from build123d import *

# Parameters (mm, degrees)
SKETCH_1_R          = 2
EXTRUDE_1_DEPTH     = 5
EXTRUDE_2_DEPTH     = 5
CUT_EXTRUDE_1_DEPTH = 6
EXTRUDE_3_DEPTH     = 5
FILLET_1_R          = 10
FILLET_2_R          = 2
SKETCH_6_R          = 2
CUT_EXTRUDE_2_DEPTH = 6


with BuildPart() as part:
    # 草图1 → 凸台-拉伸1 (new body)
    with BuildSketch(Plane(origin=(0, 0, 0), x_dir=(1, 0, 0), z_dir=(0, 1, 0))):
        with BuildLine():
            ThreePointArc((-20.0875, 4), (-23.044826598, 2.693365811), (-24.070081176, -0.372890305))
            ThreePointArc((-24.070081176, -0.372890305), (-22.780865811, -2.957326598), (-20.0875, -4))
            ThreePointArc((-20.0875, -4), (-17.130173402, -2.693365811), (-16.104918824, 0.372890305))
            Line((-16.104918824, 0.372890305), (-16.444526225, 4))
            Line((-16.444526225, 4), (-20.0875, 4))
        make_face()
        with Locations((-20.0875, 0)):
            Circle(SKETCH_1_R, mode=Mode.SUBTRACT)
        with BuildLine():
            Line((-27.14754486, 32.495352138), (-24.070081176, -0.372890305))
            ThreePointArc((-24.070081176, -0.372890305), (-23.044826598, 2.693365811), (-20.0875, 4))
            Line((-20.0875, 4), (-16.444526225, 4))
            Line((-16.444526225, 4), (-18.333300994, 24.172685504))
            Line((-18.333300994, 24.172685504), (-25.585127327, 29.683464909))
            ThreePointArc((-25.585127327, 29.683464909), (-26.661456606, 30.925425609), (-27.14754486, 32.495352138))
        make_face()
        with BuildLine():
            ThreePointArc((-20.74480004, 36.053019976), (-25.107780517, 36.364735365), (-27.14754486, 32.495352138))
            ThreePointArc((-27.14754486, 32.495352138), (-26.661456606, 30.925425609), (-25.585127327, 29.683464909))
            Line((-25.585127327, 29.683464909), (-18.333300994, 24.172685504))
            Line((-18.333300994, 24.172685504), (-19.182382508, 33.241132747))
            ThreePointArc((-19.182382508, 33.241132747), (-19.668470762, 34.811059276), (-20.74480004, 36.053019976))
        make_face()
        with Locations((-23.164963684, 32.868242443)):
            Circle(SKETCH_1_R, mode=Mode.SUBTRACT)
        with BuildLine():
            Line((22.507663644, 3.184777534), (-20.74480004, 36.053019976))
            ThreePointArc((-20.74480004, 36.053019976), (-19.668470762, 34.811059276), (-19.182382508, 33.241132747))
            Line((-19.182382508, 33.241132747), (-18.333300994, 24.172685504))
            Line((-18.333300994, 24.172685504), (8.212637649, 4))
            Line((8.212637649, 4), (20.0875, 4))
            ThreePointArc((20.0875, 4), (21.364388771, 3.790719598), (22.507663644, 3.184777534))
        make_face()
        with BuildLine():
            ThreePointArc((-16.104918824, 0.372890305), (-17.130173402, -2.693365811), (-20.0875, -4))
            Line((-20.0875, -4), (20.0875, -4))
            ThreePointArc((20.0875, -4), (18.810611229, -3.790719598), (17.667336356, -3.184777534))
            Line((17.667336356, -3.184777534), (8.212637649, 4))
            Line((8.212637649, 4), (-16.444526225, 4))
            Line((-16.444526225, 4), (-16.104918824, 0.372890305))
        make_face()
        with BuildLine():
            ThreePointArc((17.667336356, -3.184777534), (18.810611229, -3.790719598), (20.0875, -4))
            ThreePointArc((20.0875, -4), (23.878219598, -1.276888771), (22.507663644, 3.184777534))
            ThreePointArc((22.507663644, 3.184777534), (21.364388771, 3.790719598), (20.0875, 4))
            Line((20.0875, 4), (8.212637649, 4))
            Line((8.212637649, 4), (17.667336356, -3.184777534))
        make_face()
        with Locations((20.0875, 0)):
            Circle(SKETCH_1_R, mode=Mode.SUBTRACT)
        Polygon((-18.333300994, 24.172685504), (-16.444526225, 4), (8.212637649, 4), align=None)
    extrude(amount=EXTRUDE_1_DEPTH)

    # 草图2 → 凸台-拉伸2 (add)
    with BuildSketch(Plane(origin=(0, 5, 0), x_dir=(1, 0, 0), z_dir=(0, 1, 0))):
        with BuildLine():
            ThreePointArc((-20.0875, -4), (-22.780865811, -2.957326598), (-24.070081176, -0.372890305))
            Line((-24.070081176, -0.372890305), (-23.720962628, -4.10158193))
            ThreePointArc((-23.720962628, -4.10158193), (-22.290826699, -6.808468121), (-19.365512753, -7.711274824))
            Line((-19.365512753, -7.711274824), (20.460368699, -3.982583199))
            ThreePointArc((20.460368699, -3.982583199), (20.274137625, -3.995643427), (20.0875, -4))
            Line((20.0875, -4), (-20.0875, -4))
        make_face()
    extrude(amount=-EXTRUDE_2_DEPTH)

    # 草图3 → 切除-拉伸1 (cut, through all)
    with BuildSketch(Plane(origin=(0, 5, 0), x_dir=(1, 0, 0), z_dir=(0, 1, 0))):
        with BuildLine():
            ThreePointArc((-36.289327432, 17.433897667), (-37.629570165, 14.285674695), (-36.182704661, 11.185007239))
            ThreePointArc((-36.182704661, 11.185007239), (-31.653466249, 15.823666602), (-25.858788976, 18.731049718))
            Line((-25.858788976, 18.731049718), (-26.257218708, 22.986399698))
            ThreePointArc((-26.257218708, 22.986399698), (-31.612650276, 20.82332613), (-36.289327432, 17.433897667))
        make_face()
        with BuildLine():
            ThreePointArc((-25.858788976, 18.731049718), (-11.47348363, 17.605644606), (-1.756724615, 6.938492183))
            ThreePointArc((-1.756724615, 6.938492183), (0.40025314, 9.594618202), (-0.134776474, 12.974159854))
            ThreePointArc((-0.134776474, 12.974159854), (-11.569633945, 22.223545124), (-26.257218708, 22.986399698))
            Line((-26.257218708, 22.986399698), (-25.858788976, 18.731049718))
        make_face()
        with BuildLine():
            ThreePointArc((-7.176914189, 8.395044611), (-4.745829362, 6.62850376), (-1.756724615, 6.938492183))
            ThreePointArc((-1.756724615, 6.938492183), (-11.47348363, 17.605644606), (-25.858788976, 18.731049718))
            Line((-25.858788976, 18.731049718), (-25.456435977, 14.433798061))
            ThreePointArc((-25.456435977, 14.433798061), (-15.256790284, 14.622730376), (-7.176914189, 8.395044611))
        make_face()
        with BuildLine():
            ThreePointArc((-25.858788976, 18.731049718), (-31.653466249, 15.823666602), (-36.182704661, 11.185007239))
            ThreePointArc((-36.182704661, 11.185007239), (-33.358528619, 10.15793874), (-30.571035397, 11.280757314))
            ThreePointArc((-30.571035397, 11.280757314), (-28.168999159, 13.109133127), (-25.456435977, 14.433798061))
            Line((-25.456435977, 14.433798061), (-25.858788976, 18.731049718))
        make_face()
    extrude(amount=-CUT_EXTRUDE_1_DEPTH, mode=Mode.SUBTRACT)

    # 草图4 → 凸台-拉伸3 (add)
    with BuildSketch(Plane(origin=(0, 5, 0), x_dir=(1, 0, 0), z_dir=(0, 1, 0))):
        with BuildLine():
            Line((-3.809557715, 23.183657097), (8.427670456, 13.884390694))
            ThreePointArc((8.427670456, 13.884390694), (3.907166054, 20.637032025), (-3.809557715, 23.183657097))
        make_face()
    extrude(amount=-EXTRUDE_3_DEPTH)

    # 圆角1
    fillet_1_edges = [part.edges().sort_by_distance(p)[0] for p in [
        (8.427670456, 2.5, -13.884390694),
        (-3.809557715, 2.5, -23.183657097),
    ]]
    fillet(fillet_1_edges, radius=FILLET_1_R)

    # 圆角2
    fillet_2_edges = [part.edges().sort_by_distance(p)[0] for p in [
        (-26.257218708, 2.5, -22.986399698),
        (-25.456435977, 2.5, -14.433798061),
    ]]
    fillet(fillet_2_edges, radius=FILLET_2_R)

    # 草图6 → 切除-拉伸2 (cut, through all)
    with BuildSketch(Plane(origin=(0, 5, 0), x_dir=(1, 0, 0), z_dir=(0, 1, 0))):
        with Locations((-7.292808957, -2.56347694)):
            Circle(SKETCH_6_R)
    extrude(amount=-CUT_EXTRUDE_2_DEPTH, mode=Mode.SUBTRACT)


solid = part.part
Geometry check sheet. Reference: the model listing, model coordinates, mm. A direction names the side the tool comes from. Give positions to 0.01 mm unless a question says otherwise; leave off trailing zeros. Loops run counter-clockwise (first coordinate to the right, second up) from the corner with the lowest first, then second, coordinate; pieces in that order, holes last. Notation, with made-up numbers: (-8.75, -13) -> (24.25, -13) arc R15 cw to (24.25, -9) -> close; hole circle Ø9 at (63.5, -31.75). An arc over 180 degrees is marked (long way). Answer in a Markdown table with one row per item. Add a question column.
1) Cross-section at C-C on z = -27.5. Record the boundary of the cut face in (x, y).
2) Draft check along X on faces 1 (the face through (-8, 0, -5)), 2 (the face through (-4.035, 2.465, -23.719)), 3 (the face through (-10.387, 2.535, -21.733)). Enter one of: pulls with the +X half, pulls with the -X half, needs draft (parallel to the pull), parting line crosses it, or undercut.
3) Gauge pin test, flat ends, axial feed: P1, Ø3.5, axis at x = -20.09, z = 0, coming from the +Y side; P2, Ø1, axis at y = 1.5, z = -12.5, coming from the +X side. Record the tip position at first contact, or that the pin passes through.
4) Cross-section at B-B on x = 13.5. Record the boundary of the cut face in (y, z).
5) Set-up check for faces 4 (the face through (-14.563, 2.535, -14.375)), 5 (the face through (-24.956, 2.465, -14.147)), 6 (the face through (9.004, 2.465, -13.811)): record each of +Z, -Z, +X, -X, +Y, -Y from which the full face is reachable in a straight line by a thin tool's end or side.
6) Material ranges on probe 1 along X at (y, z) = (0.4, 0) (1 decimal); probe 2 along X at (y, z) = (0.65, -1.5); probe 3 along Z at (x, y) = (-6.5, 1.2), recorded low to high. Write a range as from..to.
7) Cross-section at A-A on y = 1.3. Record the boundary of the cut face in (x, z).
Outcome:
| question | item | result |
|---|---|---|
| 1 | outline | (-26.68, 0) -> (-9.49, 0) -> (-9.49, 5) -> (-26.68, 5) -> close |
| 2 | face 1 | needs draft |
| 2 | face 2 | pulls with the +X half |
| 2 | face 3 | undercut |
| 3 | P1 | passes through |
| 3 | P2 | stops at x = 10.91 |
| 4 | outline | (0, -10.03) -> (5, -10.03) -> (5, 4.63) -> (0, 4.63) -> close |
| 5 | face 4 | +Y, -Y |
| 5 | face 5 | -X, +Y, -Y |
| 5 | face 6 | -Z, +X, +Y, -Y |
| 6 | probe 1 | x = -24.1..-22.1, -18.1..18.1, 22.1..24.1 |
| 6 | probe 2 | x = -24.25..-21.41, -18.76..18.76, 21.41..23.8 |
| 6 | probe 3 | z = -25.23..-19.54, -7.59..0.73, 4.4..6.51 |
| 7 | outline | (-27.15, -32.5) arc R4 ccw to (-20.74, -36.05) -> (-6.11, -24.93) arc R10 cw to (-1.66, -23.02) arc R12.5 ccw to (7.7, -15.91) arc R10 cw to (10.73, -12.13) -> (22.51, -3.18) arc R4 ccw to (20.46, 3.98) -> (-19.37, 7.71) arc R4 ccw to (-23.72, 4.1) -> (-25.31, -12.82) arc R2 ccw to (-23.8, -14.95) arc R15.4 ccw to (-7.18, -8.4) arc R4.2 cw to (-0.13, -12.97) arc R23.8 cw to (-24.14, -23.45) arc R2 ccw to (-26.47, -25.24) -> close; hole circle Ø4 at (-23.16, -32.87); hole circle Ø4 at (-20.09, 0); hole circle Ø4 at (-7.29, 2.56); hole circle Ø4 at (20.09, 0) |
